Input: part model. Units: mm. Frame: model coordinates. A direction names the side the tool comes from. Give positions to 0.01 mm unless a question says otherwise; leave off trailing zeros. Loops run counter-clockwise (first coordinate to the right, second up) from the corner with the lowest first, then second, coordinate; pieces in that order, holes last.
from build123d import *

# Parameters (mm, degrees)
SKETCH_1_W          = 13.4
SKETCH_1_H          = 22.2
EXTRUDE_1_DEPTH     = 6.4
SKETCH_2_W          = 5
SKETCH_2_H          = 9
CUT_EXTRUDE_1_DEPTH = 6.4
SKETCH_3_W          = 3
SKETCH_3_H          = 6.2
EXTRUDE_2_DEPTH     = 9.8
SKETCH_4_R          = 2.15
CUT_EXTRUDE_2_DEPTH = 9.8


with BuildPart() as part:
    # 草图1 → 凸台-拉伸1 (new body)
    with BuildSketch(Plane.XY):
        with Locations((6.7, 11.1)):
            Rectangle(SKETCH_1_W, SKETCH_1_H)
    extrude(amount=EXTRUDE_1_DEPTH)

    # 草图2 → 切除-拉伸1 (cut)
    with BuildSketch(Plane.XY.offset(6.4)):
        with Locations((6.7, 17.7)):
            Rectangle(SKETCH_2_W, SKETCH_2_H)
    extrude(amount=-CUT_EXTRUDE_1_DEPTH, mode=Mode.SUBTRACT)

    # 草图3 → 凸台-拉伸2 (add)
    with BuildSketch(Plane.XY.offset(6.4)):
        with Locations((11.9, 6.3)):
            Rectangle(SKETCH_3_W, SKETCH_3_H)
    extrude_2 = extrude(amount=EXTRUDE_2_DEPTH)

    # 镜向1: 凸台-拉伸2 across plane
    add(extrude_2.mirror(Plane(origin=(0, 0, 3.2), x_dir=(1, 0, 0), z_dir=(0, 0, -1))))

    # 草图4 → 切除-拉伸2 (cut)
    with BuildSketch(Plane.ZY.offset(-10.4)):
        with Locations((-6.3, 6.3)):
            Circle(SKETCH_4_R)
        with Locations((12.7, 6.3)):
            Circle(SKETCH_4_R)
    extrude(amount=-CUT_EXTRUDE_2_DEPTH, mode=Mode.SUBTRACT)


solid = part.part
(1) Reachability of faces 4 (the flat face through (10.4, 6, 10)), 5 (the flat face through (12, 3.2, -5)), 6 (the flat face through (12, 9.4, 11)), 7 (the flat face through (10.4, 6, -4)) from +Z, -Z, +X, -X, +Y, -Y: full face, straight path, thin tool, end or side. Return the list, or none.
Values follow:
face 4: +Z, -X, +Y, -Y
face 5: -Z, +X, -X, -Y
face 6: +Z, +X, -X, +Y
face 7: -Z, -X, +Y, -Y
(2) Ray query, probe 1 along X at (y, z) = (17.5, 0.5); probe 2 along Y at (x, z) = (12.3, -6.3); probe 3 along X at (y, z) = (8.5, -6). Return the intervals inside material, ascending.
Values follow:
probe 1: x = 0 to 4.2, 9.2 to 13.4
probe 2: y = 3.2 to 4.15, 8.45 to 9.4
probe 3: x = 10.4 to 13.4
(3) Cut plane D-D (z = 2.5). Return the cut outline in (x, y), and give its area (3 significant figures).
Values follow:
outline: (0, 0) - (13.4, 0) - (13.4, 22.2) - (9.2, 22.2) - (9.2, 13.2) - (4.2, 13.2) - (4.2, 22.2) - (0, 22.2) - close
area: 252 mm2
(4) Cut plane C-C (y = 6.3). Return the cut outline in (x, z).
Values follow:
outline: (0, 0) - (10.4, 0) - (10.4, -4.15) - (13.4, -4.15) - (13.4, 10.55) - (10.4, 10.55) - (10.4, 6.4) - (0, 6.4) - close; (10.4, -9.8) - (13.4, -9.8) - (13.4, -8.45) - (10.4, -8.45) - close; (10.4, 14.85) - (13.4, 14.85) - (13.4, 16.2) - (10.4, 16.2) - close
(5) Cut plane A-A (z = 12.7). Return the cut outline in (x, y).
Values follow:
outline: (10.4, 3.2) - (13.4, 3.2) - (13.4, 4.15) - (10.4, 4.15) - close; (10.4, 8.45) - (13.4, 8.45) - (13.4, 9.4) - (10.4, 9.4) - close
(6) Mould query, pull axis Y, two halves, no side actions, for faces 1 (the cylindrical face through (11.88, 8.11, -5.14)), 2 (the flat face through (2, 22.2, 3)), 3 (the flat face through (13.4, 8, 3)). Classes: +Y half, -Y half, draft (parallel to the pull), parting line (faces both ways), or undercut.
Values follow:
face 1: undercut
face 2: +Y half
face 3: draft
(7) Cut plane B-B (y = 15.5). Return the cut outline in (x, z), and give its area (3 significant figures).
Values follow:
outline: (0, 0) - (4.2, 0) - (4.2, 6.4) - (0, 6.4) - close; (9.2, 0) - (13.4, 0) - (13.4, 6.4) - (9.2, 6.4) - close
area: 53.8 mm2
(8) Pin query (flat end, axial travel): pin 1 Ø2.5 at (x, z) = (12.5, 13.5) entering from -Y; pin 2 Ø1.5 at (x, z) = (11, 11) entering from +Y; pin 3 Ø5.5 at (y, z) = (6.3, -6.3) entering from -X. Return the tip coordinate at first contact, or that it passes through.
Values follow:
pin 1: stops at y = 3.2
pin 2: stops at y = 9.4
pin 3: stops at x = 10.4
